Autodesk Inventor part; units mm, degrees
ref_plane "Work Plane1" through (0, -62.5, 0) normal (0, 1, 0) x (-1, 0, 0)
ref_plane "YZ Plane" through (0, 0, 0) normal (1, 0, 0) x (0, 1, 0)
ref_plane "XY Plane" through (0, 0, 0) normal (0, 0, 1) x (1, 0, 0)
sketch "Sketch1" plane through (0, 0, 0) normal (0, 1, 0) x (-1, 0, 0)
  line L0 (0, 0) -> (42, 0)
  line L1 (42, 0) -> (42, -42)
  line L2 (42, -42) -> (0, -42)
  line L3 (0, -42) -> (0, 0)
  line L4 (0, 0) -> (42, 0)
  line L5 (42, 0) -> (42, -42)
  line L6 (42, -42) -> (0, -42)
  line L7 (0, -42) -> (0, 0)
  line L8 (42, -21) -> (42, -5.25)
  circle A0 centre (36.75, -5.25) radius 1.5
  circle A1 centre (36.75, -36.75) radius 1.5
  circle A2 centre (5.25, -36.75) radius 1.5
  circle A3 centre (5.25, -5.25) radius 1.5
  dimension "d0" = 42
  dimension "d1" = 42
  dimension "d2" = 3
  dimension "d3" = 3
  dimension "d4" = 3
  dimension "d5" = 3
extrude "Extrusion1" add sketch "Sketch1" along normal blind 5 and the other way blind 2.5
sketch "Sketch2" plane through (0, 5, 0) normal (0, 1, 0) x (1, 0, 0)
  circle A0 centre (-21, 21) radius 11.5
  point P0 (0, 0)
  point P1 (-42, 0)
  dimension "d9" = 23
extrude "Extrusion2" cut sketch "Sketch2" against normal up to surface (7.5 mm away)
sketch "Sketch3" plane through (0, 5, 0) normal (0, 1, 0) x (1, 0, 0)
  circle A0 centre (-21, 21) radius 11.5
  circle A1 centre (-21, 21) radius 13.5
  circle A2 centre (-21, 21) radius 3.5
  point P0 (0, 0)
  dimension "d12" = 27
  dimension "d13" = 7
extrude "Extrusion3" add sketch "Sketch3" along normal blind 3 contours A0 | A1
sketch "Sketch4" plane through (-42, -2.5, 0) normal (0, 0, 1) x (1, 0, 0)
  line L0 (42, 7.5) -> (42, 2.5)
  line L1 (42, 7.5) -> (0.1256, 7.5)
  line L2 (42, -112.5) -> (42, 7.5)
  line L3 (42, -112.5) -> (42, -122.5)
  line L4 (42, -132.5) -> (42, -122.5)
  line L5 (0, 0) -> (0, 7.5)
  line L6 (42, -132.5) -> (0, -132.5)
  line L7 (0, -132.5) -> (0, 7.5)
  line L8 (0, 7.5) -> (42, 7.5)
  line L9 (42, 7.5) -> (42, -132.5)
  point P0 (0.1256, 7.5)
  dimension "d20" = 10
extrude "Extrusion4" add sketch "Sketch4" along normal blind 6
ref_plane "Work Plane1" through (0, -62.5, 0) normal (0, 1, 0) x (-1, 0, 0)
ref_plane "Work Plane3" through (0, -65, 0) normal (0, 1, 0) x (1, 0, 0)
mirror "Mirror5" about plane through (0, -65, 0) normal (0, 1, 0) of "Extrusion1", "Extrusion3", "Extrusion2"
sketch "Sketch8" plane through (0, -2.5, -42) normal (1, 0, 0) x (0, 0, -1)
  line L0 (0, 7.5) -> (0, 0)
  line L1 (-48, -132.5) -> (-48, 7.5)
  line L2 (0, 7.5) -> (-48, 7.5)
  line L3 (-48, 7.5) -> (-48, -132.5)
  line L4 (-48, -132.5) -> (0, -132.5)
  line L5 (0, -132.5) -> (0, 7.5)
  line L6 (0, 0) -> (-42, 0)
  line L7 (-21.0744, 0) -> (-42, -20.9256)
  line L8 (-42, -125) -> (-42, 2.5)
  line L9 (-21.0744, 0) -> (8.5189, 0) construction
  line L10 (0, 0) -> (-42, 0)
  line L11 (-42, -20.9256) -> (-42, 2.5)
  line L12 (0, 7.5) -> (0, 0)
  line L13 (-21.0744, 0) -> (0, 0)
  line L14 (-42, -20.9256) -> (-42, -132.5)
  line L15 (0, -132.5) -> (-48, -132.5)
  line L16 (0, 0) -> (0, -2)
  line L17 (0, -2) -> (-21.0744, -2)
  line L18 (-21.0744, -2) -> (-21.0744, 0)
  line L19 (-21.0744, -2) -> (-42, -23)
  line L20 (-42, -23) -> (-40, -23)
  line L21 (-40.0407, -21.0337) -> (-40.0407, -130.0337)
  line L22 (-40.0407, -130.0337) -> (-40.0407, -132.5)
  dimension "d64" = 135
  dimension "d67" = 2
extrude "Extrusion8" add sketch "Sketch8" along normal blind 4 contours L0 L6 L8 L14 L4 L1 L2 | L5 L17 L18 L6 | L7 L8 L6 | L18 L19 L8 L7 | L14 L8 L20 L21 L22 L4 | L21 L20 L19
mirror "Mirror6" about plane through (0, -65, 0) normal (0, 1, 0) of "Extrusion8"
ref_plane "Work Plane4" through (-21, -2.5, -42) normal (-1, 0, 0) x (0, 0, 1)
mirror "Mirror7" about plane through (-21, -2.5, -42) normal (-1, 0, 0) of "Extrusion8", "Mirror6"
sketch "Sketch9" plane through (0, -4.5, -42) normal (0, 0, -1) x (-1, 0, 0)
  line L0 (-4, 9.5) -> (-4, -130.5)
  line L1 (-4, 9.5) -> (-0.25, 9.5)
  line L2 (-0.25, 9.5) -> (-0.25, 5.75)
  line L3 (-0.25, 5.75) -> (-4, 5.75)
  line L4 (-4, 5.75) -> (-4, 9.5)
  line L5 (-4, -130.5) -> (46, -130.5)
  line L6 (46, -130.5) -> (42.25, -130.5)
  line L7 (42.25, -130.5) -> (42.25, -126.75)
  line L8 (42.25, -126.75) -> (46, -126.75)
  line L9 (46, -126.75) -> (46, -130.5)
  circle A0 centre (-0.25, 5.75) radius 1.5
  circle A1 centre (42.25, -126.75) radius 1.5
  circle A2 centre (42.25, 5.75) radius 1.5
  circle A3 centre (-0.25, -126.75) radius 1.5
  point P0 (0, 4.5)
  dimension "d71" = 3.75
  dimension "d72" = 3.75
  dimension "d73" = 3.75
  dimension "d74" = 3.75
  dimension "d75" = 3
  dimension "d76" = 3
  dimension "d77" = 3
  dimension "d78" = 3
extrude "Extrusion9" cut sketch "Sketch9" against normal blind 15 contours A0 L2 L3 | L3 L2 A0 | A1 L8 L7 | L7 L8 A1 | A2 | A3
thread "Thread5"
thread "Thread6"
thread "Thread7"
thread "Thread8"
thread "Thread9"
thread "Thread10"
thread "Thread11"
thread "Thread12"
thread "Thread13"
thread "Thread14"
thread "Thread15"
thread "Thread16"
fillet "Fillet1" radius 1 1 edges at (-32.5, 5, -21)
fillet "Fillet2" radius 1 1 edges at (-32.5, -135, -21)
properties part number "stepperMotorLink"
Can you work these out from the model? Positions are in its coordinate system, mm. A direction names the side the tool comes from. Coordinates: 2 decimals unless noted, no trailing zeros. Write each loop counter-clockwise with the first axis right and the second up, starting at its lowest first coordinate (ties: lowest second). Pieces come first, ordered by that corner, then holes.
Q1. For P1, Ø3.5, axis at x = -5.25, z = -36.75, coming from the -Y side; P2, Ø6, axis at x = -23.5, y = -17, coming from the -Z side; P3, Ø3.5, axis at x = -5.25, z = -5.25, coming from the +Y side, each with a flat end and sliding along its axis, tell me the tip position at first contact or that it passes through.
Results found:
P1: stops at y = -135
P2: stops at z = 0
P3: stops at y = 5
Q2. Imagine slicing it at D-D, the plane y = -51.5. List the corners of the cut face in (x, z) for me.
Results found:
outline: (-46, -1.96) - (-42, -1.96) - (-42, 0) - (0, 0) - (0, -1.96) - (4, -1.96) - (4, 6) - (-46, 6) - close
Q3. Imagine slicing it at C-C, the plane z = -36.75. Count the separate pieces of the cut face and the enclosed holes in it, plus the area to 3 significant figures.
Results found:
separate pieces: 6
enclosed holes: 4
area: 664 mm2
Q4. Which directions (+Z, -Z, +X, -X, +Y, -Y) give clear straight access to the entire face, cutting with the end or side of a thin tool? Please do faces 4 (the face through (-44, -4.5, -31)), 5 (the face through (-42, -70, -1)), 6 (the face through (-16, 5, -21)).
Results found:
face 4: -Z, +X, -X
face 5: -Z
face 6: none
Q5. If we mould it in two halves opening along X, with no side actions, what happens to faces 1 (the face through (-8.123, -136.479, -25.055)), 2 (the face through (-43.97, -116.12, -11.58)), 3 (the face through (-42, -131, -27))? For each: +X half, -X half, draft (parallel to the pull), parting line (faces both ways), or undercut.
Results found:
face 1: parting line
face 2: draft
face 3: undercut
Q6. Imagine slicing it at B-B, the plane y = -131.25. List the corners of the cut face in (x, z) for me, plus the area to 3 significant figures.
Results found:
outline: (-46, -42) - (-43.75, -42) - (-43.75, -27) - (-40.75, -27) - (-40.75, -42) - (-1.25, -42) - (-1.25, -27) - (1.75, -27) - (1.75, -42) - (4, -42) - (4, 6) - (-46, 6) - close; hole circle Ø3 at (-36.75, -36.75); hole circle Ø3 at (-36.75, -5.25); hole circle Ø23 at (-21, -21); hole circle Ø3 at (-5.25, -36.75); hole circle Ø3 at (-5.25, -5.25)
area: 1,870 mm2
Q7. Imagine slicing it at A-A, the plane x = -36.75. List the corners of the cut face in (y, z) for me, plus the area to 3 significant figures.
Results found:
outline: (-135, -42) - (-127.5, -42) - (-127.5, -38.25) - (-135, -38.25) - close; (-135, -35.25) - (-127.5, -35.25) - (-127.5, -6.75) - (-135, -6.75) - close; (-135, -3.75) - (-127.5, -3.75) - (-127.5, 0) - (-2.5, 0) - (-2.5, -3.75) - (5, -3.75) - (5, 6) - (-135, 6) - close; (-2.5, -42) - (5, -42) - (5, -38.25) - (-2.5, -38.25) - close; (-2.5, -35.25) - (5, -35.25) - (5, -6.75) - (-2.5, -6.75) - close
area: 1,380 mm2
Q8. Please list where these lines run through material, in increasing order: L1, parallel to Y at x = 0.25, z = -39; L2, parallel to X at y = -132, z = -5; L3, parallel to Z at x = -21, y = -136.35.
Results found:
L1: y = -135 to -132.75, -129.75 to -125.5, -4.5 to -0.25, 2.75 to 5
L2: x = -46 to -38.23, -35.27 to -6.73, -3.77 to 4
L3: z = -34.5 to -24.5, -17.5 to -7.5
